from build123d import *

# Parameters (mm, degrees)
SKETCH1_R           = 19.05
BOSS_EXTRUDE1_DEPTH = 6.604
FILLET1_R           = 12.7
FILLET2_R           = 8.89


with BuildPart() as part:
    # Sketch1 → Boss-Extrude1 (new body)
    with BuildSketch(Plane.XY):
        with BuildLine():
            Line((-31.115, 165.1), (31.115, 165.1))
            Line((31.115, 165.1), (61.595, 130.81))
            Line((61.595, 130.81), (77.47, 102.87))
            Line((77.47, 102.87), (35.853421773, -12.889613927))
            ThreePointArc((35.853421773, -12.889613927), (0, -38.1), (-35.853421773, -12.889613927))
            Line((-35.853421773, -12.889613927), (-77.47, 102.87))
            Line((-77.47, 102.87), (-61.595, 130.81))
            Line((-61.595, 130.81), (-31.115, 165.1))
        make_face()
        Circle(SKETCH1_R, mode=Mode.SUBTRACT)
    extrude(amount=BOSS_EXTRUDE1_DEPTH)

    # Fillet1
    fillet1_edges = [part.edges().sort_by_distance(p)[0] for p in [
        (61.595, 130.81, 3.302),
        (77.47, 102.87, 3.302),
        (-77.47, 102.87, 3.302),
        (-61.595, 130.81, 3.302),
    ]]
    fillet(fillet1_edges, radius=FILLET1_R)

    # Fillet2
    fillet2_edges = [part.edges().sort_by_distance(p)[0] for p in [
        (-31.115, 165.1, 3.302),
        (31.115, 165.1, 3.302),
    ]]
    fillet(fillet2_edges, radius=FILLET2_R)


solid = part.part
Model file for the job. Use its own axes, mm. Give positions to 0.01 mm unless a question says otherwise; leave off trailing zeros. Write each loop counter-clockwise with the first axis right and the second up, starting at its lowest first coordinate (ties: lowest second). Pieces come first, ordered by that corner, then holes. Notation, with made-up numbers: M 20.5,11.5 L 56.5,11.5 A25 ccw 56.5,32.5 Z; hole C 72.5,76 d1. An arc over 180 degrees is marked long. One line per item, written item: value. Start each with the question number.
Q1. Two-plate mould, pull along Y, no slides. Class faces 1 (the flat face through (1, 88, 0)), 2 (the flat face through (55.95, 43.01, 3.26)), 3 (the cylindrical face through (-15.12, -11.59, 3.26)): +Y half, -Y half, draft (parallel to the pull), parting line (faces both ways), or undercut.
Q2. Saw through at A-A, the plane z = 4.75. Write the cut outline in (x, y).
Q3. Saw through at B-B, the plane x = 0. Write the cut outline in (y, z).
Q4. Drop a flat-ended pin along its axis: pin 1 Ø1 at (y, z) = (-17.5, 5.5) entering from -X. Give the stop position or say it passes through.
Q5. Saw through at D-D, the plane x = 55. Write the cut outline in (y, z), plus the area to 3 significant figures.
Q6. Probe probe 1 along Y at (x, z) = (0, 4.25); probe 2 along X at (y, z) = (4, 3.75); probe 3 along Y at (x, z) = (-3.5, 4.75). List the from-to ranges inside material, lowest first. Write a range as [from, to].
Q7. Saw through at C-C, the plane y = 0. Write the cut outline in (x, z).
Output values:
1. face 1: draft
1. face 2: -Y half
1. face 3: undercut
2. outline: M -75.49,97.38 L -35.85,-12.89 A38.1 ccw 35.85,-12.89 L 75.49,97.38 A12.7 ccw 74.59,107.95 L 62.26,129.65 A12.7 ccw 60.71,131.81 L 33.77,162.12 A8.89 ccw 27.12,165.1 L -27.12,165.1 A8.89 ccw -33.77,162.12 L -60.71,131.81 A12.7 ccw -62.26,129.65 L -74.59,107.95 A12.7 ccw Z; hole C 0,0 d38.1
3. outline: M -38.1,0 L -19.05,0 L -19.05,6.6 L -38.1,6.6 Z; M 19.05,0 L 165.1,0 L 165.1,6.6 L 19.05,6.6 Z
4. pin 1: stops at x = -34.1
5. outline: M 40.37,0 L 138.23,0 L 138.23,6.6 L 40.37,6.6 Z
5. area: 646 mm²
6. probe 1: y = [-38.1, -19.05], [19.05, 165.1]
6. probe 2: x = [-41.93, -18.63], [18.63, 41.93]
6. probe 3: y = [-37.94, -18.73], [18.73, 165.1]
7. outline: M -40.49,0 L -19.05,0 L -19.05,6.6 L -40.49,6.6 Z; M 19.05,0 L 40.49,0 L 40.49,6.6 L 19.05,6.6 Z
